from build123d import *

# Parameters (mm, degrees)
SKETCH1_W           = 285
SKETCH1_H           = 260
BOSS_EXTRUDE3_DEPTH = 5
SKETCH3_W           = 259
SKETCH3_H           = 236
BOSS_EXTRUDE4_DEPTH = 20
SKETCH4_W           = 249
SKETCH4_H           = 226
CUT_EXTRUDE1_DEPTH  = 20


with BuildPart() as part:
    # Sketch1 → Boss-Extrude3 (new body)
    with BuildSketch(Plane.XY):
        with Locations((20.685479664, 43.047709924)):
            Rectangle(SKETCH1_W, SKETCH1_H)
    extrude(amount=BOSS_EXTRUDE3_DEPTH)

    # Sketch3 → Boss-Extrude4 (add)
    with BuildSketch(Plane.XY.offset(5)):
        with Locations((20.685479664, 41.047709924)):
            Rectangle(SKETCH3_W, SKETCH3_H)
    extrude(amount=BOSS_EXTRUDE4_DEPTH)

    # Sketch4 → Cut-Extrude1 (cut)
    with BuildSketch(Plane.XY.offset(25)):
        with Locations((20.685479664, 41.047709924)):
            Rectangle(SKETCH4_W, SKETCH4_H)
    extrude(amount=-CUT_EXTRUDE1_DEPTH, mode=Mode.SUBTRACT)


solid = part.part
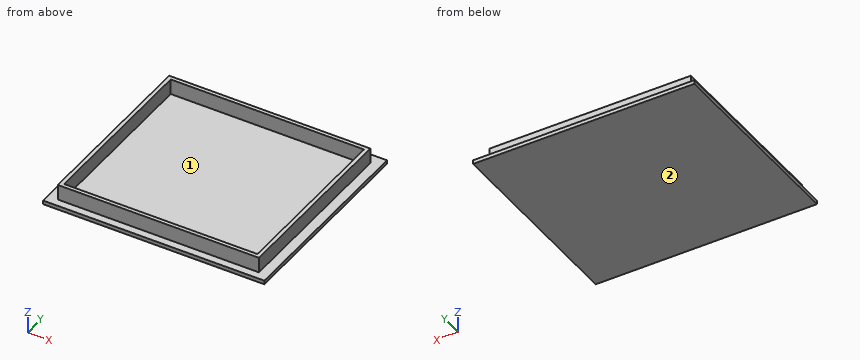
Read the model definition and answer for the solid it produces. Units are mm, in the model's axes. Face numbers are marked on the shaded views. Round coordinates to 2 decimals unless told otherwise and drop trailing zeros. Loops run counter-clockwise (first coordinate to the right, second up) from the corner with the lowest first, then second, coordinate; pieces in that order, holes last.
Q1. Section B-B on y = 1.5 is taken. Write down the section's boundary in (x, z).
Q2. Consider probe 1 along X at (y, z) = (67, 8.25); probe 2 along Y at (x, z) = (-45, 16); probe 3 along Z at (x, y) = (80.5, -64.5). Determine where each line is inside the solid, lowest interval first.
Q3. Determine the mould class of the marked faces 1 and 2 for opening direction X: released by +X, released by -X, zero draft, split by the parting line, or undercut.
Q4. Section A-A on z = 11.25 is taken. Write down the section's boundary in (x, y).
Q5. Section C-C on x = -40 is taken. Write down the section's boundary in (y, z), and give its area (3 significant figures).
Q6. Each of these flat-tipped pins is pushed along its axis until it touches: pin 1 (3 mm diameter, centred on y = 2.5, z = 13, fed in from +X); pin 2 (2 mm diameter, centred on y = -33, z = 15.5, fed in from -X); pin 3 (5 mm diameter, centred on x = -4.5, z = 17, fed in from -Y); pin 4 (6 mm diameter, centred on y = 65, z = 7.5, fed in from +X). Where does it stop, or does it pass through?
Output:
1. outline: (-121.81, 0) - (163.19, 0) - (163.19, 5) - (150.19, 5) - (150.19, 25) - (145.19, 25) - (145.19, 5) - (-103.81, 5) - (-103.81, 25) - (-108.81, 25) - (-108.81, 5) - (-121.81, 5) - close
2. probe 1: x = -108.81 to -103.81, 145.19 to 150.19
2. probe 2: y = -76.95 to -71.95, 154.05 to 159.05
2. probe 3: z = 0 to 5
3. face 1: undercut
3. face 2: zero draft
4. outline: (-108.81, -76.95) - (150.19, -76.95) - (150.19, 159.05) - (-108.81, 159.05) - close; hole (-103.81, -71.95) - (145.19, -71.95) - (145.19, 154.05) - (-103.81, 154.05) - close
5. outline: (-86.95, 0) - (173.05, 0) - (173.05, 5) - (159.05, 5) - (159.05, 25) - (154.05, 25) - (154.05, 5) - (-71.95, 5) - (-71.95, 25) - (-76.95, 25) - (-76.95, 5) - (-86.95, 5) - close
5. area: 1,500 mm2
6. pin 1: stops at x = 150.19
6. pin 2: stops at x = -108.81
6. pin 3: stops at y = -76.95
6. pin 4: stops at x = 163.19
